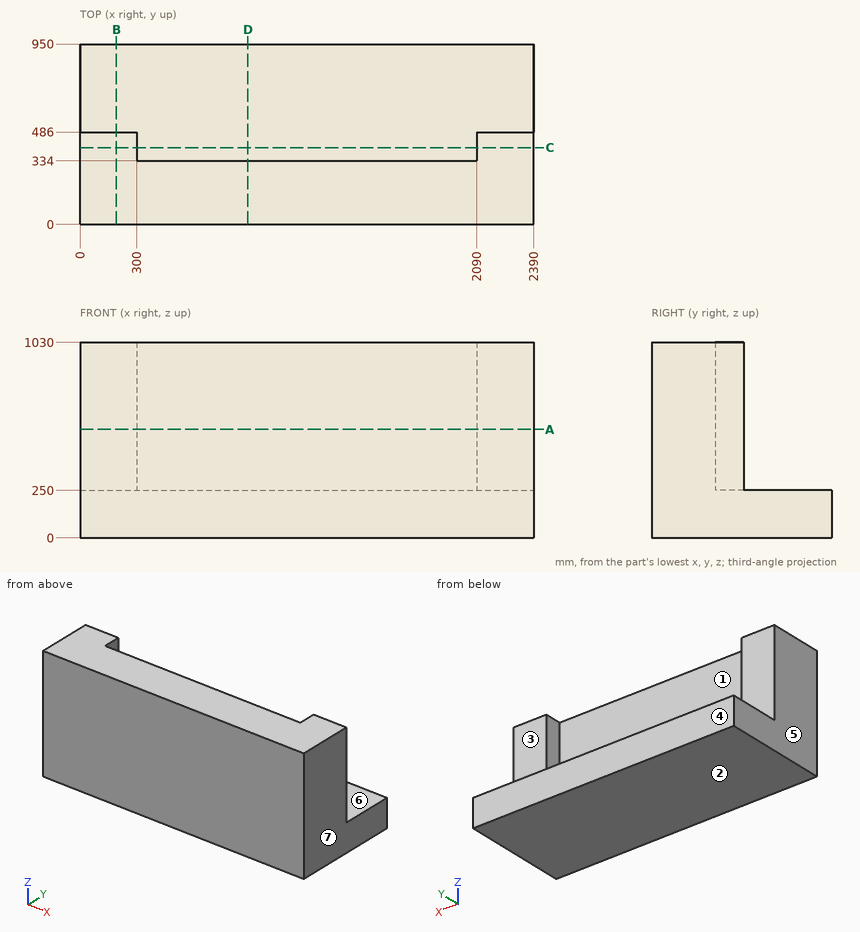
Drawing for the job (mm, zero at the part's lowest x, y, z). A direction names the side the tool comes from. Coordinates: 2 decimals unless noted, no trailing zeros. Write each loop counter-clockwise with the first axis right and the second up, starting at its lowest first coordinate (ties: lowest second). Pieces come first, ordered by that corner, then holes. Notation, with made-up numbers: (87.25, 61) - (130.25, 61) arc R25 ccw to (130.25, 95) - close; hole circle Ø10 at (33, 43.5). An arc over 180 degrees is marked (long way). Write each question's results on one line, items separated by ' | '. Start each with the question number.
1) Probe line 1 along X through (y, z) = (403, 453); line 2 along Z through (x, y) = (1223.5, 627); line 3 along Y through (x, z) = (1400.5, 360). List the from-to ranges inside material, lowest first. Write a range as from..to.
2) 3-axis set-ups, long thin cutter, end or side, ignore diameter. For the marked faces 1, 2 and 3: which of +Z, -Z, +X, -X, +Y, -Y reach the whole face in a straight line?
3) Flat gauge pins, fed straight in: P1, Ø8, axis at x = 1311, z = 248, coming from the -Y side; P2, Ø3, axis at x = 755, y = 588, coming from the +Z side. Where does each tip first touch, or does it go through?
4) Mould opens along X. For the marked faces 4, 5, 6 and 7 say: pulls with the +X half, pulls with the -X half, needs draft (parallel to the pull), parting line crosses it, or undercut.
5) Cut at B-B (x = 191). Write the cut outline in (y, z), then the cut area to 3 significant figures.
6) Cut at C-C (y = 404). Write the cut outline in (x, z), then the cut area to 3 significant figures.
7) Cut at A-A (z = 572). Write the cut outline in (x, y), then the cut area to 3 significant figures.
8) Cut at D-D (x = 884.5). Write the cut outline in (y, z), then the cut area to 3 significant figures.
Returned:
1) line 1: 0..300, 2090..2390 | line 2: 0..250 | line 3: 0..334
2) face 1: +Z, +Y | face 2: -Z, +X, -X, +Y, -Y | face 3: +Z, +X, -X, +Y
3) P1: y = 0 | P2: z = 250
4) face 4: needs draft | face 5: pulls with the -X half | face 6: undercut | face 7: pulls with the +X half
5) outline: (0, 0) - (950, 0) - (950, 250) - (486, 250) - (486, 1030) - (0, 1030) - close | area: 617,000 mm^2
6) outline: (0, 0) - (2390, 0) - (2390, 1030) - (2090, 1030) - (2090, 250) - (300, 250) - (300, 1030) - (0, 1030) - close | area: 1,070,000 mm^2
7) outline: (0, 0) - (2390, 0) - (2390, 486) - (2090, 486) - (2090, 334) - (300, 334) - (300, 486) - (0, 486) - close | area: 889,000 mm^2
8) outline: (0, 0) - (950, 0) - (950, 250) - (334, 250) - (334, 1030) - (0, 1030) - close | area: 498,000 mm^2
